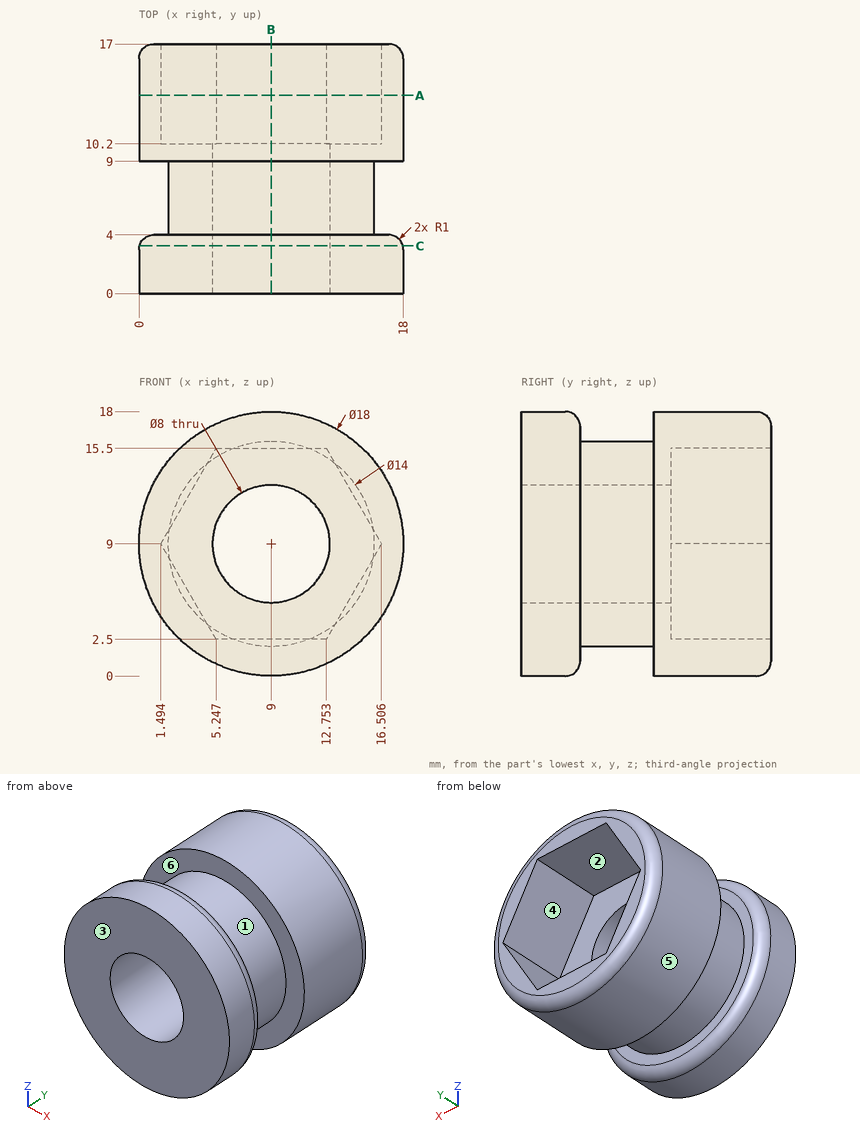
Drawing for the job (mm, zero at the part's lowest x, y, z). A direction names the side the tool comes from. Round coordinates to 2 decimals unless told otherwise and drop trailing zeros. Loops run counter-clockwise (first coordinate to the right, second up) from the corner with the lowest first, then second, coordinate; pieces in that order, holes last. Notation, with made-up numbers: (27.5, -19) -> (71.5, -19) arc R25 cw to (71.5, 16) -> close; hole circle Ø6 at (-23, -29). An arc over 180 degrees is marked (long way). Answer in a Markdown table with one row per item.
Item 1: Which spindle directions (+Z, -Z, +X, -X, +Y, -Y) get a long thin tool onto all of the face, cutting with end or side? Do the marked faces 4, 5 and 6. Say none if no direction does.
Answers below:
| item | result |
|---|---|
| face 4 | +Y |
| face 5 | +Y, -Y |
| face 6 | none |
Item 2: Pin check, flat tips, straight feed: pin 1 (1.5 mm diameter, centred on x = 7, z = 5, fed in from +Y); pin 2 (3 mm diameter, centred on y = 10.5, z = 15.5, fed in from +X); pin 3 (4 mm diameter, centred on x = 6.5, y = 5, fed in from +Z). Stop position of each tip, or through.
Answers below:
| item | result |
|---|---|
| pin 1 | stops at y = 10.2 |
| pin 2 | stops at x = 16.48 |
| pin 3 | stops at z = 17.84 |
Item 3: Saw through at B-B (x = 9). Write the cut outline in (y, z).
Answers below:
| item | result |
|---|---|
| outline | (0, 0) -> (3, 0) arc R1 ccw to (4, 1) -> (4, 2) -> (9, 2) -> (9, 0) -> (16, 0) arc R1 ccw to (17, 1) -> (17, 2.5) -> (10.2, 2.5) -> (10.2, 5) -> (0, 5) -> close; (0, 13) -> (10.2, 13) -> (10.2, 15.5) -> (17, 15.5) -> (17, 17) arc R1 ccw to (16, 18) -> (9, 18) -> (9, 16) -> (4, 16) -> (4, 17) arc R1 ccw to (3, 18) -> (0, 18) -> close |
Item 4: Mould opens along Z. For the marked faces 1, 2 and 3 say: +Z half, -Z half, draft (parallel to the pull), parting line (faces both ways), or undercut.
Answers below:
| item | result |
|---|---|
| face 1 | parting line |
| face 2 | undercut |
| face 3 | draft |
Item 5: Saw through at A-A (y = 13.5). Write the cut outline in (x, z) (1 decimal).
Answers below:
| item | result |
|---|---|
| outline | circle Ø18 at (9, 9); hole (1.5, 9) -> (5.2, 2.5) -> (12.8, 2.5) -> (16.5, 9) -> (12.8, 15.5) -> (5.2, 15.5) -> close |
Item 6: Drill centre lines: L1, parallel to Y at x = 15.5, z = 5.5; L2, parallel to X at y = 5, z = 9; L3, parallel to Y at x = 8.5, z = 3. Where is each one in solid material? Low to high. Write a range as [from, to].
Answers below:
| item | result |
|---|---|
| L1 | y = [0, 4], [9, 17] |
| L2 | x = [2, 5], [13, 16] |
| L3 | y = [0, 10.2] |
Item 7: Saw through at C-C (y = 3.25). Write the cut outline in (x, z).
Answers below:
| item | result |
|---|---|
| outline | circle Ø17.94 at (9, 9); hole circle Ø8 at (9, 9) |
